Here's how the part is built. I have some questions about the finished solid (model axes, mm). A direction names the side the tool comes from. Coordinates: 2 decimals unless noted, no trailing zeros. Order: outer loops, then holes, each group sorted by start corner. A loop starts at its lowest first (then second) coordinate and runs counter-clockwise, first axis right, second up.
Autodesk Inventor part; units mm, degrees
ref_plane "YZ Plane" through (0, 0, 0) normal (1, 0, 0) x (0, 1, 0)
ref_plane "XZ Plane" through (0, 0, 0) normal (0, 1, 0) x (-1, 0, 0)
ref_plane "XY Plane" through (0, 0, 0) normal (0, 0, 1) x (1, 0, 0)
sketch "Sketch1" plane through (0, 0, 0) normal (0, 1, 0) x (-1, 0, 0)
  circle A0 centre (0, 0) radius 8
  dimension "d0" = 16
extrude "Extrusion1" add sketch "Sketch1" along normal blind 7.1
sketch "Sketch2" plane through (0, 7.1, 0) normal (0, 1, 0) x (1, 0, 0)
  circle A0 centre (0, 0) radius 6
  dimension "d3" = 12
extrude "Extrusion2" add sketch "Sketch2" along normal blind 7.4
sketch "Sketch3" plane through (0, 14.5, 0) normal (0, 1, 0) x (1, 0, 0)
  circle A0 centre (0, 0) radius 8
extrude "Extrusion3" add sketch "Sketch3" along normal blind 1.5
chamfer "Chamfer1" distance 0.5 angle 45 4 edges at (-8, 16, 0) (-8, 14.5, 0) (8, 7.1, 0) (8, 0, 0)
sketch "Sketch4" plane through (0, 16, 0) normal (0, 1, 0) x (1, 0, 0)
  circle A0 centre (0, 0) radius 3
  dimension "d11" = 6
extrude "Extrusion4" cut sketch "Sketch4" against normal blind 16
properties part number "2GT_wheel"
Q1. Will these pins go through, and if not, where does the flat tip stop? pin 1 (8 mm diameter, centred on x = -5.5, z = 3, fed in from -Y); pin 2 (3 mm diameter, centred on y = 12, z = -0.5, fed in from -X); pin 3 (1.5 mm diameter, centred on x = -3, y = 7, fed in from -Z); pin 4 (4 mm diameter, centred on x = -6, y = 7, fed in from -Z).
Q2. I need wall thicknesses on L1, parallel to X at y = 8, z = 0; L2, parallel to Y at x = -5, z = -4.25. Which ranges of each line are inside material? Lowest first, please.
Q3. For faces 1 (the flat face through (0.1, 0, -3.2)), 2 (the flat face through (2, 14.5, -6)), which set-ups out of +Z, -Z, +X, -X, +Y, -Y let a thin tool reach every point of the face, with its end or its side?
Q4. We'd pull the mould along Z, two halves only. Please class faces 3 (the flat face through (-2, 7.1, 6)), 4 (the cylindrical face through (-3, 8, 0)), 5 (the cylindrical face through (-6, 11, 0)): pulls with the +Z half, pulls with the -Z half, needs draft (parallel to the pull), parting line crosses it, or undercut.
Q5. If we section it at C-C on y = 10.25: Write out the boundary of the cut face in (x, z).
Q6. If we section it at A-A on z = 0: Write out the boundary of the cut face in (x, y), then the cut area to 3 significant figures.
Q7. If we section it at B-B on x = 0: Write out the boundary of the cut face in (y, z).
Q8. If we section it at D-D on y = 5.5: Write out the boundary of the cut face in (x, z), then the cut area to 3 significant figures.
Reply:
1. pin 1: stops at y = 0
1. pin 2: stops at x = -6
1. pin 3: stops at z = -7.64
1. pin 4: stops at z = -6.9
2. L1: x = -6 to -3, 3 to 6
2. L2: y = 0 to 7.1, 14.5 to 16
3. face 1: +Z, -Z, +X, -X, -Y
3. face 2: none
4. face 3: needs draft
4. face 4: undercut
4. face 5: parting line crosses it
5. outline: circle Ø12 at (0, 0); hole circle Ø6 at (0, 0)
6. outline: (-8, 0.5) - (-7.5, 0) - (-3, 0) - (-3, 16) - (-7.5, 16) - (-8, 15.5) - (-8, 15) - (-7.5, 14.5) - (-6, 14.5) - (-6, 7.1) - (-7.5, 7.1) - (-8, 6.6) - close; (3, 0) - (7.5, 0) - (8, 0.5) - (8, 6.6) - (7.5, 7.1) - (6, 7.1) - (6, 14.5) - (7.5, 14.5) - (8, 15) - (8, 15.5) - (7.5, 16) - (3, 16) - close
6. area: 129 mm2
7. outline: (0, -7.5) - (0.5, -8) - (6.6, -8) - (7.1, -7.5) - (7.1, -6) - (14.5, -6) - (14.5, -7.5) - (15, -8) - (15.5, -8) - (16, -7.5) - (16, -3) - (0, -3) - close; (0, 3) - (16, 3) - (16, 7.5) - (15.5, 8) - (15, 8) - (14.5, 7.5) - (14.5, 6) - (7.1, 6) - (7.1, 7.5) - (6.6, 8) - (0.5, 8) - (0, 7.5) - close
8. outline: circle Ø16 at (0, 0); hole circle Ø6 at (0, 0)
8. area: 173 mm2
